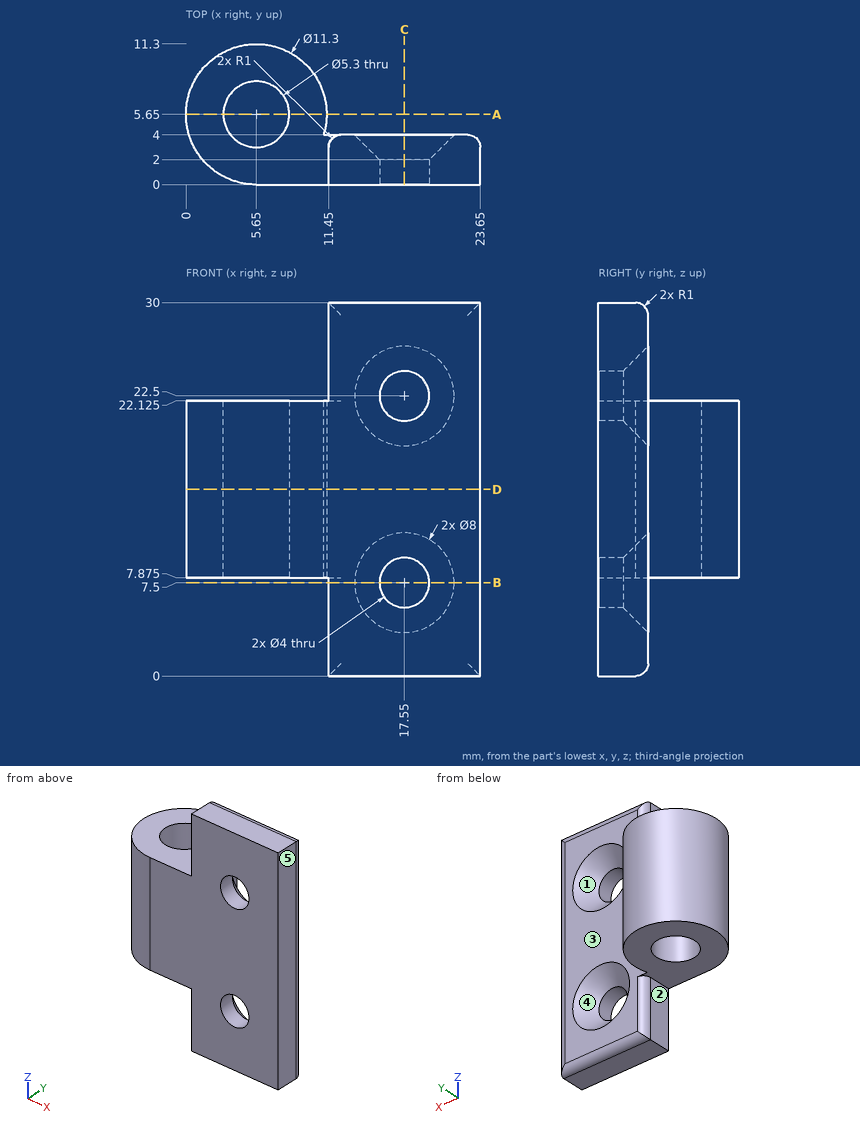
Can you work these out from the drawing? Everything is in mm from the part's minimum corner. A direction names the side the tool comes from. Give positions to 0.01 mm unless a question says otherwise; leave off trailing zeros. Order: outer loops, then holes, each group sorted by start corner. A loop starts at its lowest first (then second) coordinate and runs counter-clockwise, first axis right, second up.
Item 1: If we section it at A-A, the plane y = 5.65: Write out the boundary of the cut face in (x, z) (3 decimals), plus the area to 3 significant figures.
Item 2: If we section it at D-D, the plane z = 15: Write out the boundary of the cut face in (x, y), plus the area to 3 significant figures.
Item 3: If we section it at C-C, the plane x = 17.55: Write out the boundary of the cut face in (y, z), plus the area to 3 significant figures.
Item 4: I need wall thicknesses on line 1 (Z direction, x = 17.55, y = 0.55); line 2 (X direction, y = 1.4, z = 7.5); line 3 (Y direction, x = 5.65, z = 14.75). Which ranges of each line are inside material? Lowest first, please.
Item 5: If we mould it in two halves opening along X, with no side actions, what happens to the marked faces 3, 4 and 5? For each: pulls with the +X half, pulls with the -X half, needs draft (parallel to the pull), parting line crosses it, or undercut.
Item 6: For the marked faces 1 and 2, which set-ups out of +Z, -Z, +X, -X, +Y, -Y let a thin tool reach every point of the face, with its end or its side?
Item 7: I'm going to push flat-ended pins straight in: pin 1 (4 mm diameter, centred on x = 20, y = 7, fed in from +Z); pin 2 (2.5 mm diameter, centred on y = 2, z = 28, fed in from -X); pin 3 (4 mm diameter, centred on x = 3, z = 14.5, fed in from -Y); pin 4 (3 mm diameter, centred on x = 4, y = 5, fed in from -Z) (3 decimals). Where does each tip first touch, or does it pass through?
Item 8: If we section it at B-B, the plane z = 7.5: Write out the boundary of the cut face in (x, y).
Values:
1. outline: (0, 7.875) - (3, 7.875) - (3, 22.125) - (0, 22.125) - close; (8.3, 7.875) - (11.3, 7.875) - (11.3, 22.125) - (8.3, 22.125) - close
1. area: 85.5 mm2
2. outline: (5.65, 0) - (23.65, 0) - (23.65, 3) arc R1 ccw to (22.65, 4) - (11.05, 4) arc R5.65 ccw (long way) to start; hole circle Ø5.3 at (5.65, 5.65)
2. area: 134 mm2
3. outline: (0, 0) - (3, 0) arc R1 ccw to (4, 1) - (4, 3.5) - (2, 5.5) - (0, 5.5) - close; (0, 9.5) - (2, 9.5) - (4, 11.5) - (4, 18.5) - (2, 20.5) - (0, 20.5) - close; (0, 24.5) - (2, 24.5) - (4, 26.5) - (4, 29) arc R1 ccw to (3, 30) - (0, 30) - close
3. area: 79.6 mm2
4. line 1: z = 0 to 5.5, 9.5 to 20.5, 24.5 to 30
4. line 2: x = 11.45 to 15.55, 19.55 to 23.65
4. line 3: y = 0 to 3, 8.3 to 11.3
5. face 3: needs draft
5. face 4: undercut
5. face 5: pulls with the +X half
6. face 1: +Y
6. face 2: -Z, -X, +Y, -Y
7. pin 1: passes through
7. pin 2: stops at x = 11.45
7. pin 3: stops at y = 0.04
7. pin 4: stops at z = 7.875
8. outline: (11.45, 0) - (15.55, 0) - (15.55, 2) - (13.55, 4) - (12.45, 4) arc R1 ccw to (11.45, 3) - close; (19.55, 0) - (23.65, 0) - (23.65, 3) arc R1 ccw to (22.65, 4) - (21.55, 4) - (19.55, 2) - close
